from build123d import *

# Parameters (mm, degrees)
SKETCH1_R           = 1.6
BOSS_EXTRUDE1_DEPTH = 0.5


with BuildPart() as part:
    # Sketch1 → Boss-Extrude1 (new body, symmetric)
    with BuildSketch(Plane(origin=(0, 0, 0), x_dir=(0, 0, -1), z_dir=(1, 0, 0))):
        with BuildLine():
            Line((-10, 4), (-6, 4))
            ThreePointArc((-6, 4), (-4.585786438, 4.585786438), (-4, 6))
            Line((-4, 6), (-4, 12))
            ThreePointArc((-4, 12), (0, 16), (4, 12))
            Line((4, 12), (4, 6))
            ThreePointArc((4, 6), (4.585786438, 4.585786438), (6, 4))
            Line((6, 4), (10, 4))
            ThreePointArc((10, 4), (14, 0), (10, -4))
            Line((10, -4), (-10, -4))
            ThreePointArc((-10, -4), (-14, 0), (-10, 4))
        make_face()
        with Locations((0, 12)):
            Circle(SKETCH1_R, mode=Mode.SUBTRACT)
        with BuildLine():
            Line((-10, 1.6), (10, 1.6))
            ThreePointArc((10, 1.6), (11.6, 0), (10, -1.6))
            Line((10, -1.6), (-10, -1.6))
            ThreePointArc((-10, -1.6), (-11.6, 0), (-10, 1.6))
        make_face(mode=Mode.SUBTRACT)
    extrude(amount=BOSS_EXTRUDE1_DEPTH, both=True)


solid = part.part
The listing builds one solid part. Answer for the finished solid, in the listing's coordinates (mm). A direction names the side the tool comes from. Coordinates: 2 decimals unless noted, no trailing zeros. Write each loop counter-clockwise with the first axis right and the second up, starting at its lowest first coordinate (ties: lowest second). Pieces come first, ordered by that corner, then holes. Notation, with made-up numbers: (35.25, -3) - (47.25, -3) arc R13 ccw to (47.25, 19) - close; hole circle Ø8 at (61, -38.75). An arc over 180 degrees is marked (long way). Return JSON: item names as keys, results as strings.
1. The part is cut by section C-C on z = 7.75. Determine the outline of the cut face in (x, y).
Final values:
{"outline": "(-0.5, -4) - (0.5, -4) - (0.5, -1.6) - (-0.5, -1.6) - close; (-0.5, 1.6) - (0.5, 1.6) - (0.5, 4) - (-0.5, 4) - close"}
2. The part is cut by section A-A on y = 0. Determine the outline of the cut face in (x, z).
Final values:
{"outline": "(-0.5, -14) - (0.5, -14) - (0.5, -11.6) - (-0.5, -11.6) - close; (-0.5, 11.6) - (0.5, 11.6) - (0.5, 14) - (-0.5, 14) - close"}
3. Consider line 1 along Y through (x, z) = (-0.1, 0); line 2 along Y through (x, z) = (-0.05, 9.75); line 3 along Y through (x, z) = (0.2, -5). Determine where each line is inside the solid, lowest interval first.
Final values:
{"line 1": "-4 to -1.6, 1.6 to 10.4, 13.6 to 16", "line 2": "-4 to -1.6, 1.6 to 4", "line 3": "-4 to -1.6, 1.6 to 4.27"}
4. The part is cut by section D-D on z = 0. Determine the outline of the cut face in (x, y).
Final values:
{"outline": "(-0.5, -4) - (0.5, -4) - (0.5, -1.6) - (-0.5, -1.6) - close; (-0.5, 1.6) - (0.5, 1.6) - (0.5, 10.4) - (-0.5, 10.4) - close; (-0.5, 13.6) - (0.5, 13.6) - (0.5, 16) - (-0.5, 16) - close"}
5. This flat-tipped pin is pushed along its axis until it touches: pin 1 Ø0.5 at (x, y) = (0, 8.5) entering from +Z. Where does it stop, or does it pass through?
Final values:
{"pin 1": "z = 4"}
6. Which of the six approach directions +Z, -Z, +X, -X, +Y, -Y give full straight-line access (tool end or side, diameter ignored) to faces 1 (the face through (0, 0, 14)), 2 (the face through (0, 4, -8)), 3 (the face through (0, 0, 11.6)), 4 (the face through (0, 4, 8))?
Final values:
{"face 1": "+Z, +X, -X", "face 2": "-Z, +X, -X, +Y", "face 3": "+X, -X", "face 4": "+Z, +X, -X, +Y"}
7. For a pull along Z with two mould halves and no side action, classify faces 5 (the face through (-0.007, 13.586, 0.208)), 6 (the face through (0, -4, 0)), 7 (the face through (0, 9, -4)) as +Z half, -Z half, draft (parallel to the pull), parting line (faces both ways), or undercut.
Final values:
{"face 5": "undercut", "face 6": "draft", "face 7": "-Z half"}
8. The part is cut by section B-B on x = -0.05. Determine the outline of the cut face in (y, z).
Final values:
{"outline": "(-4, -10) arc R4 ccw to (4, -10) - (4, -6) arc R2 cw to (6, -4) - (12, -4) arc R4 ccw to (12, 4) - (6, 4) arc R2 cw to (4, 6) - (4, 10) arc R4 ccw to (-4, 10) - close; hole (-1.6, -10) arc R1.6 ccw to (1.6, -10) - (1.6, 10) arc R1.6 ccw to (-1.6, 10) - close; hole circle Ø3.2 at (12, 0)"}
